The model under review builds one solid part; all positions refer to its coordinate system, in mm. A direction names the side the tool comes from. Round coordinates to 2 decimals unless told otherwise and drop trailing zeros. Write each loop counter-clockwise with the first axis right and the second up, starting at its lowest first coordinate (ties: lowest second). Pieces come first, ordered by that corner, then holes. Notation, with made-up numbers: (44, 69) - (93, 69) arc R18 ccw to (93, 90) - close; hole circle Ø8 at (61, 58.25). An arc over 180 degrees is marked (long way). Write each question's results on one line, items separated by ' | '.
```python
from build123d import *

# Parameters (mm, degrees)
SKETCH_1_R               = 14
EXTRUDE_1_DEPTH          = 3.5
SKETCH_2_R               = 6
EXTRUDE_2_DEPTH          = 11.5
SKETCH_3_R               = 3
CUT_EXTRUDE_1_DEPTH      = 25.839484697
SKETCH_4_R               = 1.55
CUT_EXTRUDE_2_DEPTH      = 23.896506284
PATTERN_CIRCULAR_1_COUNT = 4
PATTERN_CIRCULAR_2_COUNT = 2
PATTERN_CIRCULAR_2_ANGLE = 90


with BuildPart() as part:
    # 草图1 → 凸台-拉伸1 (new body)
    with BuildSketch(Plane.XY):
        Circle(SKETCH_1_R)
    extrude(amount=EXTRUDE_1_DEPTH)

    # 草图2 → 凸台-拉伸2 (add)
    with BuildSketch(Plane.XY.offset(3.5)):
        Circle(SKETCH_2_R)
    extrude(amount=EXTRUDE_2_DEPTH)

    # 草图3 → 切除-拉伸1 (cut, through all)
    with BuildSketch(Plane.XY.offset(15)):
        Circle(SKETCH_3_R)
    extrude(amount=-CUT_EXTRUDE_1_DEPTH, mode=Mode.SUBTRACT)

    # 草图4 → 切除-拉伸2 (cut, through all)
    with BuildSketch(Plane.XY.offset(3.5)):
        with Locations((0, 10)):
            Circle(SKETCH_4_R)
    cut_extrude_2 = extrude(amount=-CUT_EXTRUDE_2_DEPTH, mode=Mode.SUBTRACT)

    # 阵列(圆周)1: 切除-拉伸2 ×4 about axis
    pattern_circular_1_axis = Axis((0, 0, 0), (0, 0, 1))
    for i in range(1, PATTERN_CIRCULAR_1_COUNT):
        add(cut_extrude_2.rotate(pattern_circular_1_axis, i * 360 / PATTERN_CIRCULAR_1_COUNT), mode=Mode.SUBTRACT)

    # 草图6 → M3 螺纹孔1 (revolve, cut)
    with BuildSketch(Plane(origin=(0, 0, 9), x_dir=(0, 0, 1), z_dir=(0, 1, 0))):
        Polygon((0, 0), (0, 8.251075774), (1.25, 7.5), (1.25, 0.275), (1.525, 0), align=None)
    hole_wizard_m3_1 = revolve(axis=Axis((-6.35, 0, 9), (1, 0, 0)), mode=Mode.SUBTRACT)

    # 阵列(圆周)2: M3 螺纹孔1 ×2 about axis
    pattern_circular_2_axis = Axis((0, 0, 15), (0, 0, 1))
    for i in range(1, PATTERN_CIRCULAR_2_COUNT):
        add(hole_wizard_m3_1.rotate(pattern_circular_2_axis, i * PATTERN_CIRCULAR_2_ANGLE / (PATTERN_CIRCULAR_2_COUNT - 1)), mode=Mode.SUBTRACT)


solid = part.part
```
Q1. We need section A-A (x = 0). State the section outline as (y, z) points, plus the area to 3 significant figures.
Evaluation:
outline: (-14, 0) - (-11.55, 0) - (-11.55, 3.5) - (-14, 3.5) - close; (-8.45, 0) - (-3, 0) - (-3, 15) - (-6, 15) - (-6, 3.5) - (-8.45, 3.5) - close; (3, 0) - (8.45, 0) - (8.45, 3.5) - (6, 3.5) - (6, 7.75) - (3, 7.75) - close; (3, 10.25) - (6, 10.25) - (6, 15) - (3, 15) - close; (11.55, 0) - (14, 0) - (14, 3.5) - (11.55, 3.5) - close | area: 117 mm^2
Q2. For probe 1 along Y at (x, z) = (0, 2.8); probe 2 along Z at (x, y) = (13.25, 3.5); probe 3 along Z at (x, y) = (5.35, 0), list the stretches that pass through material, from the lowest coordinate up.
Evaluation:
probe 1: y = -14 to -11.55, -8.45 to -3, 3 to 8.45, 11.55 to 14 | probe 2: z = 0 to 3.5 | probe 3: z = 0 to 7.75, 10.25 to 15
Q3. We need section D-D (x = 10). State the section outline as (y, z) points.
Evaluation:
outline: (-9.8, 0) - (-1.55, 0) - (-1.55, 3.5) - (-9.8, 3.5) - close; (1.55, 0) - (9.8, 0) - (9.8, 3.5) - (1.55, 3.5) - close
Q4. We need section C-C (z = 3). State the section outline as (x, y) points.
Evaluation:
outline: circle Ø28 at (0, 0); hole circle Ø3.1 at (-10, 0); hole circle Ø6 at (0, 0); hole circle Ø3.1 at (0, -10); hole circle Ø3.1 at (0, 10); hole circle Ø3.1 at (10, 0)
Q5. Insertion check: P1, Ø2, axis at y = 0, z = 9, coming from the +X side; P2, Ø4, axis at x = 0, y = 10, coming from the +Z side; P3, Ø3, axis at x = 0, y = -10, coming from the +Z side; P4, Ø2, axis at x = 3.5, z = 3.5, coming from the +Y side (3 decimals). Each pin has a flat end and moves straight along its axis. Give the tip position at first contact, or say it passes through.
Evaluation:
P1: stops at x = -2.83 | P2: stops at z = 3.5 | P3: passes through | P4: stops at y = 13.775
Q6. The part is to be moulded in two halves that separate along Z. For faces 1 (the cylindrical face through (4.34, -1.24, 8.84)), 2 (the cylindrical face through (-0.336, 8.487, 1.774)), 3 (the flat face through (6, -3, 3.5)), say which applies: released by +Z, released by -Z, zero draft, split by the parting line, or undercut.
Evaluation:
face 1: undercut | face 2: zero draft | face 3: released by +Z
Q7. Tool access review of faces 4 (the cylindrical face through (-2.4, -1.8, 7.6)), 5 (the cylindrical face through (-1.301, -5.857, 9.17)), 6 (the cylindrical face through (1.24, 4.34, 8.84)): name each direction out of +Z, -Z, +X, -X, +Y, -Y from which nothing blocks a thin tool from reaching the whole face with its end or side.
Evaluation:
face 4: +Z, -Z | face 5: +Z | face 6: +Y
